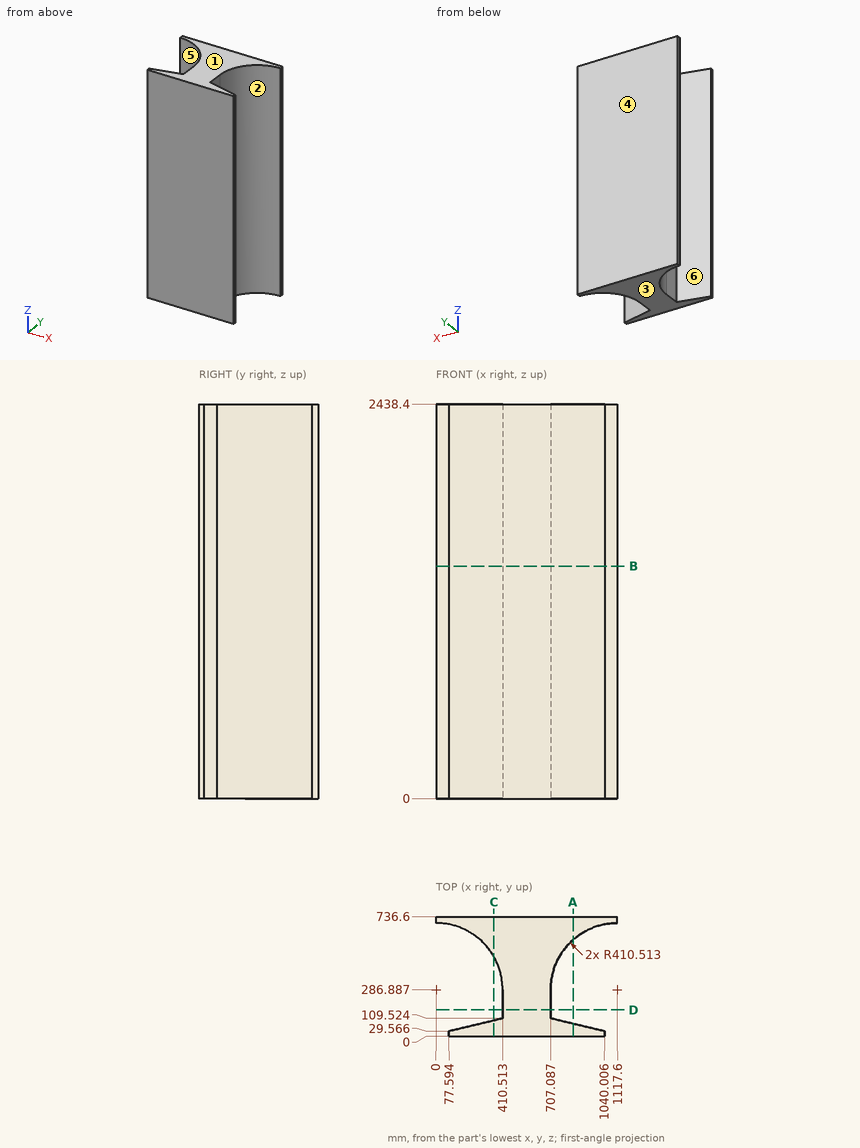
The drawing under review shows one solid part. Ordinate dimensions are in mm from its lowest x, y, z. A direction names the side the tool comes from. Round coordinates to 2 decimals unless told otherwise and drop trailing zeros. Write each loop counter-clockwise with the first axis right and the second up, starting at its lowest first coordinate (ties: lowest second). Pieces come first, ordered by that corner, then holes. Notation, with made-up numbers: (67, -39.75) - (77, -39.75) arc R24 cw to (77, -10.75) - close; hole circle Ø10 at (18, 7). An arc over 180 degrees is marked (long way). Use a Markdown table: item, result. Add a question column.
1. We need section D-D (y = 162). State the section outline as (x, z) points.
2. We need section C-C (x = 356). State the section outline as (y, z) points.
3. Wall thickness on probe 1 along X at (y, z) = (267, 1856); probe 2 along Y at (x, z) = (739, 937.5) (1 decimal); probe 3 along Y at (x, z) = (325.5, 1798) (1 decimal): over which ranges is each line inside the solid? List them lowest first.
4. For the marked faces 1 and 2, list the 3-axis set-ups (+Z, -Z, +X, -X, +Y, -Y) from which the entire face can be reached by the end or side of a thin tool; tool diameter is ignored.
5. We need section A-A (x = 845.5). State the section outline as (y, z) points.
6. Mouldability with a two-part tool opening along Y and no side actions: class the marked faces 3, 4, 5 and 6 as +Y half, -Y half, draft (parallel to the pull), parting line (faces both ways), or undercut.
7. We need section B-B (z = 1437). State the section outline as (x, y) points (1 decimal), then the cut area to 3 significant figures.
8. Clearance check with flat-ended pins moving along their axes: pin 1 (12 mm diameter, centred on y = 213.5, z = 869.5, fed in from +X); pin 2 (8 mm diameter, centred on y = 480.5, z = 1524.5, fed in from +X); pin 3 (9 mm diameter, centred on y = 15.5, z = 1131.5, fed in from +X). State where each tip first meets the part, or that it passes through.
Output:
| question | item | result |
|---|---|---|
| 1 | outline | (410.51, 0) - (707.09, 0) - (707.09, 2438.4) - (410.51, 2438.4) - close |
| 2 | outline | (0, 0) - (96.43, 0) - (96.43, 2438.4) - (0, 2438.4) - close; (491.3, 0) - (736.6, 0) - (736.6, 2438.4) - (491.3, 2438.4) - close |
| 3 | probe 1 | x = 410.51 to 707.09 |
| 3 | probe 2 | y = 0 to 101.9, 445.6 to 736.6 |
| 3 | probe 3 | y = 0 to 89.1, 537 to 736.6 |
| 4 | face 1 | +Z, +X, -X, +Y, -Y |
| 4 | face 2 | +Z, -Z, +X |
| 5 | outline | (0, 0) - (76.28, 0) - (76.28, 2438.4) - (0, 2438.4) - close; (594.27, 0) - (736.6, 0) - (736.6, 2438.4) - (594.27, 2438.4) - close |
| 6 | face 3 | draft |
| 6 | face 4 | +Y half |
| 6 | face 5 | undercut |
| 6 | face 6 | undercut |
| 7 | outline | (0, 697.4) arc R410.5 cw to (410.5, 286.9) - (410.5, 109.5) - (77.6, 29.6) - (77.6, 0) - (1040, 0) - (1040, 29.6) - (707.1, 109.5) - (707.1, 286.9) arc R410.5 cw to (1117.6, 697.4) - (1117.6, 736.6) - (0, 736.6) - close |
| 7 | area | 369,000 mm2 |
| 8 | pin 1 | stops at x = 707.09 |
| 8 | pin 2 | stops at x = 757.78 |
| 8 | pin 3 | stops at x = 1040.01 |
